Input: dimensioned drawing with shaded views. Units: mm. Origin: part minimum x, y, z. A direction names the side the tool comes from. Give positions to 0.01 mm unless a question says otherwise; leave off trailing zeros. Loops run counter-clockwise (first coordinate to the right, second up) from the corner with the lowest first, then second, coordinate; pieces in that order, holes last.
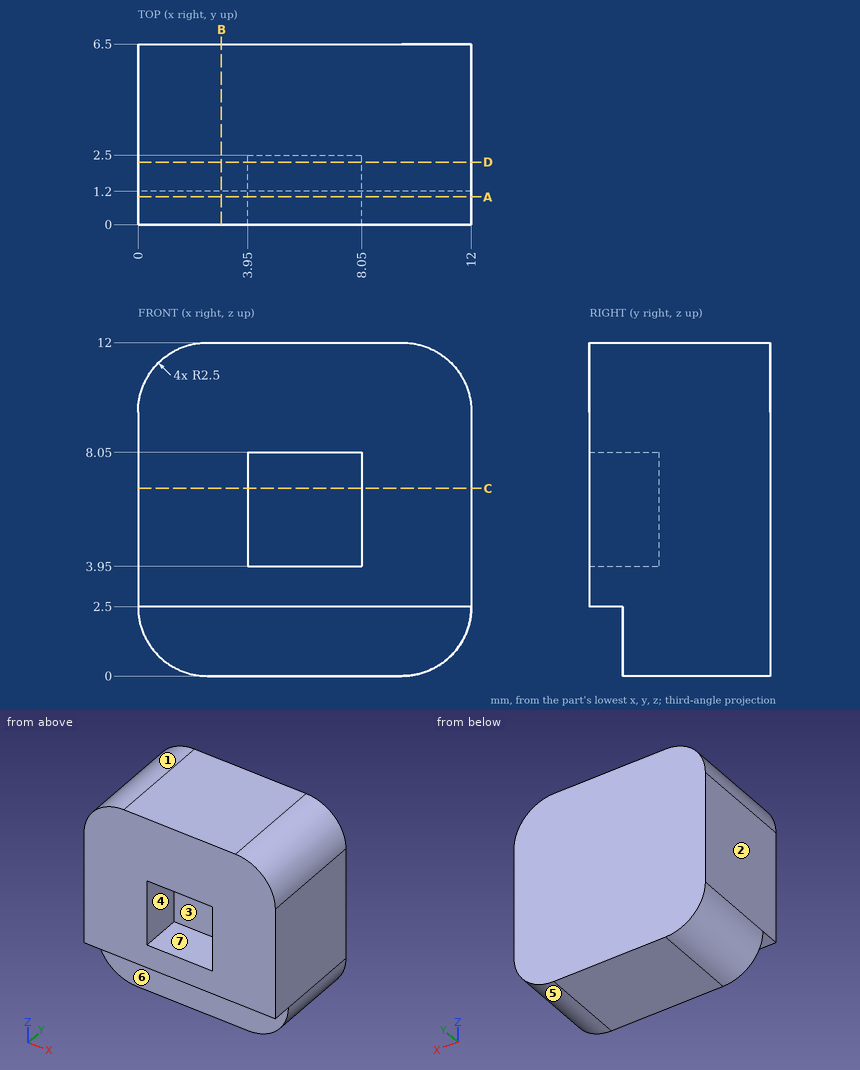
Item 1: Section query A-A on y = 1. Return loops of the section in (x, z), plus the area to 3 significant figures.
Values follow:
outline: (0, 2.5) - (12, 2.5) - (12, 9.5) arc R2.5 ccw to (9.5, 12) - (2.5, 12) arc R2.5 ccw to (0, 9.5) - close; hole (3.95, 3.95) - (8.05, 3.95) - (8.05, 8.05) - (3.95, 8.05) - close
area: 94.5 mm2
Item 2: Ray query, probe 1 along Y at (x, z) = (6, 6.5); probe 2 along Y at (x, z) = (9, 0.5); probe 3 along X at (y, z) = (1.75, 4.5). Return the intervals inside material, ascending.
Values follow:
probe 1: y = 2.5 to 6.5
probe 2: y = 1.2 to 6.5
probe 3: x = 0 to 3.95, 8.05 to 12
Item 3: Pin query (flat end, axial travel): pin 1 (1.2 mm diameter, centred on x = 4, z = 1.5, fed in from -Y); pin 2 (2 mm diameter, centred on x = 7, z = 7, fed in from -Y). Return the tip coordinate at first contact, or that it passes through.
Values follow:
pin 1: stops at y = 1.2
pin 2: stops at y = 2.5
Item 4: Section query B-B on x = 3. Return loops of the section in (y, z).
Values follow:
outline: (0, 2.5) - (1.2, 2.5) - (1.2, 0) - (6.5, 0) - (6.5, 12) - (0, 12) - close
Item 5: Draft query along Z for the marked faces 1, 2, 3 and 4. Return one class per face: +Z half, -Z half, draft (parallel to the pull), parting line (faces both ways), or undercut.
Values follow:
face 1: +Z half
face 2: draft
face 3: undercut
face 4: undercut
Item 6: Section query D-D on y = 2.25. Return loops of the section in (x, z), plus the area to 3 significant figures.
Values follow:
outline: (0, 2.5) arc R2.5 ccw to (2.5, 0) - (9.5, 0) arc R2.5 ccw to (12, 2.5) - (12, 9.5) arc R2.5 ccw to (9.5, 12) - (2.5, 12) arc R2.5 ccw to (0, 9.5) - close; hole (3.95, 3.95) - (8.05, 3.95) - (8.05, 8.05) - (3.95, 8.05) - close
area: 122 mm2
Item 7: Set-up query: the marked faces 5, 6 and 7. Return all of +Z, -Z, +X, -X, +Y, -Y with unobstructed straight access to the full face (end or side cutting, diameter ignored); none if empty.
Values follow:
face 5: -Z, +X, +Y, -Y
face 6: -Z, +X, -X, -Y
face 7: -Y
Item 8: Section query C-C on z = 6.75. Return loops of the section in (x, y), plus the area to 4 significant figures.
Values follow:
outline: (0, 0) - (3.95, 0) - (3.95, 2.5) - (8.05, 2.5) - (8.05, 0) - (12, 0) - (12, 6.5) - (0, 6.5) - close
area: 67.75 mm2
